```python
from build123d import *

# Parameters (mm, degrees)
SKETCH2_R            = 71
BOSS_EXTRUDE1_DEPTH  = 11
SKETCH12_R           = 57.5
SKETCH12_R_2         = 23.75
CUT_EXTRUDE8_DEPTH   = 1
CUT_EXTRUDE9_START   = -10
SKETCH10_R           = 85
SKETCH10_R_2         = 81
CUT_EXTRUDE9_DEPTH   = 10
SKETCH14_R           = 57.5
SKETCH14_R_2         = 23.75
BOSS_EXTRUDE2_DEPTH  = 1
SKETCH15_R           = 81
BOSS_EXTRUDE3_DEPTH  = 4
SKETCH16_R           = 57.5
SKETCH16_R_2         = 23.75
CUT_EXTRUDE11_DEPTH  = 2
SKETCH17_W           = 29
SKETCH17_H           = 10.11
SKETCH17_H_2         = 35.11
BOSS_EXTRUDE4_DEPTH  = 3
SKETCH19_R           = 80.970867582
BOSS_EXTRUDE5_DEPTH  = 2
BOSS_EXTRUDE6_START  = -3
SKETCH20_R           = 80.970867582
BOSS_EXTRUDE6_DEPTH  = 3
SKETCH21_W           = 29
SKETCH21_H           = 45.22
BOSS_EXTRUDE7_DEPTH  = 4
BOSS_EXTRUDE9_DEPTH  = 5
CUT_EXTRUDE12_START  = -5
SKETCH26_R           = 80.970867582
CUT_EXTRUDE12_DEPTH  = 5
BOSS_EXTRUDE10_START = -4
SKETCH27_R           = 80.970867582
BOSS_EXTRUDE10_DEPTH = 4
CUT_EXTRUDE15_REACH  = 120.043
SKETCH28_R           = 80.970867582
SKETCH28_R_2         = 80


with BuildPart() as part:
    # Sketch1 → Revolve1 (revolve)
    with BuildSketch(Plane.XY, mode=Mode.PRIVATE) as revolve1_sk:
        Polygon((0, 12), (0, 15), (85, 15), (85, 10.5), (84, 10.5), (77, 3.5), (77, 0), (71, 0), (71, 12), (23.75, 12), (23.75, -7.5), (21.25, -7.5), (21.25, 6), (6.5, 6), (6.5, 9), (0, 9), align=None)
    revolve(revolve1_sk.sketch.rotate(Axis((0, 12, 0), (0, -1, 0)), 180), axis=Axis((0, 12, 0), (0, -1, 0)))

    # Sketch2 → Boss-Extrude1 (add)
    with BuildSketch(Plane.XZ.offset(-12)):
        with Locations(Location((0, 0, 0), (0, 0, 180))):
            Circle(SKETCH2_R)
        Polygon((0, 70.292395274), (-60.875, 35.146197637), (-60.875, -35.146197637), (0, -70.292395274), (60.875, -35.146197637), (60.875, 35.146197637), align=None, mode=Mode.SUBTRACT)
    extrude(amount=BOSS_EXTRUDE1_DEPTH)

    # Sketch12 → Cut-Extrude8 (cut)
    with BuildSketch(Plane.XZ.offset(-12)):
        Circle(SKETCH12_R)
        with Locations(Location((0, 0, 0), (0, 0, 180))):
            Circle(SKETCH12_R_2, mode=Mode.SUBTRACT)
    extrude(amount=-CUT_EXTRUDE8_DEPTH, mode=Mode.SUBTRACT)

    # Sketch10 → Cut-Extrude9 (cut)
    with BuildSketch(Plane(origin=(0, 15, 0), x_dir=(1, 0, 0), z_dir=(0, 1, 0)).offset(CUT_EXTRUDE9_START)):
        Circle(SKETCH10_R)
        with Locations(Location((0, 0, 0), (0, 0, 180))):
            Circle(SKETCH10_R_2, mode=Mode.SUBTRACT)
    extrude(amount=CUT_EXTRUDE9_DEPTH, mode=Mode.SUBTRACT)

    # Sketch14 → Boss-Extrude2 (add)
    with BuildSketch(Plane(origin=(0, 13, 0), x_dir=(-1, 0, 0), z_dir=(0, -1, 0))):
        with Locations(Location((0, 0, 0), (0, 0, 180))):
            Circle(SKETCH14_R)
        Circle(SKETCH14_R_2, mode=Mode.SUBTRACT)
    extrude(amount=-BOSS_EXTRUDE2_DEPTH)

    # Sketch15 → Boss-Extrude3 (add)
    with BuildSketch(Plane(origin=(0, 15, 0), x_dir=(1, 0, 0), z_dir=(0, 1, 0))):
        with Locations(Location((0, 0, 0), (0, 0, 180))):
            Circle(SKETCH15_R)
    extrude(amount=BOSS_EXTRUDE3_DEPTH)

    # Sketch16 → Cut-Extrude11 (cut)
    with BuildSketch(Plane.XZ.offset(-13)):
        Circle(SKETCH16_R)
        with Locations(Location((0, 0, 0), (0, 0, 180))):
            Circle(SKETCH16_R_2, mode=Mode.SUBTRACT)
    extrude(amount=-CUT_EXTRUDE11_DEPTH, mode=Mode.SUBTRACT)

    # Sketch17 → Boss-Extrude4 (add)
    with BuildSketch(Plane(origin=(0, 19, 0), x_dir=(1, 0, 0), z_dir=(0, 1, 0))):
        with Locations((-48.833648901, -5.055)):
            Rectangle(SKETCH17_W, SKETCH17_H)
        with Locations((-48.833648901, 17.555)):
            Rectangle(SKETCH17_W, SKETCH17_H_2)
        with Locations((48.416351099, -5.055)):
            Rectangle(SKETCH17_W, SKETCH17_H)
        with Locations((48.416351099, 17.555)):
            Rectangle(SKETCH17_W, SKETCH17_H_2)
    extrude(amount=BOSS_EXTRUDE4_DEPTH)

    # Sketch19 → Boss-Extrude5 (add)
    with BuildSketch(Plane(origin=(0, 19, 0), x_dir=(1, 0, 0), z_dir=(0, 1, 0))):
        with Locations(Location((0, 0, 0), (0, 0, 180))):
            Circle(SKETCH19_R)
    extrude(amount=BOSS_EXTRUDE5_DEPTH)

    # Sketch20 → Boss-Extrude6 (add)
    with BuildSketch(Plane(origin=(0, 21, 0), x_dir=(1, 0, 0), z_dir=(0, 1, 0)).offset(BOSS_EXTRUDE6_START)):
        with Locations(Location((0, 0, 0), (0, 0, 180))):
            Circle(SKETCH20_R)
    extrude(amount=BOSS_EXTRUDE6_DEPTH)

    # Sketch21 → Boss-Extrude7 (add)
    with BuildSketch(Plane(origin=(0, 22, 0), x_dir=(1, 0, 0), z_dir=(0, 1, 0))):
        with Locations((48.416351099, 12.5)):
            Rectangle(SKETCH21_W, SKETCH21_H)
        with Locations((-48.833648901, 12.5)):
            Rectangle(SKETCH21_W, SKETCH21_H)
    extrude(amount=BOSS_EXTRUDE7_DEPTH)

    # Sketch22 → Boss-Extrude9 (add)
    with BuildSketch(Plane(origin=(0, 21, 0), x_dir=(1, 0, 0), z_dir=(0, 1, 0))):
        Polygon((48.416351099, 35.11), (37.416351099, 35.11), (37.416351099, 50.11), (59.416351099, 50.11), (59.416351099, 35.11), align=None)
    extrude(amount=BOSS_EXTRUDE9_DEPTH)

    # Sketch26 → Cut-Extrude12 (cut)
    with BuildSketch(Plane(origin=(0, 26, 0), x_dir=(1, 0, 0), z_dir=(0, 1, 0)).offset(CUT_EXTRUDE12_START)):
        with Locations(Location((0, 0, 0), (0, 0, 180))):
            Circle(SKETCH26_R)
    extrude(amount=CUT_EXTRUDE12_DEPTH, mode=Mode.SUBTRACT)

    # Sketch27 → Boss-Extrude10 (add)
    with BuildSketch(Plane(origin=(0, 21, 0), x_dir=(1, 0, 0), z_dir=(0, 1, 0)).offset(BOSS_EXTRUDE10_START)):
        with Locations(Location((0, 0, 0), (0, 0, 180))):
            Circle(SKETCH27_R)
    extrude(amount=BOSS_EXTRUDE10_DEPTH)

    # Cut-Extrude15: up to this cone (the profile starts inside it)
    cut_extrude15_end = Plane(origin=(0, 21, 0), z_dir=(0, 1, 0)).offset(-94.499999) * Cone(1e-06, 309.543, 309.542999, align=(Align.CENTER, Align.CENTER, Align.MIN), mode=Mode.PRIVATE)
    # Sketch28 → Cut-Extrude15 (cut, up to the surface)
    with BuildSketch(Plane(origin=(0, 21, 0), x_dir=(1, 0, 0), z_dir=(0, 1, 0)), mode=Mode.PRIVATE) as cut_extrude15_sk1:
        Circle(SKETCH28_R)
        with Locations(Location((0, 0, 0), (0, 0, 180))):
            Circle(SKETCH28_R_2, mode=Mode.SUBTRACT)
    cut_extrude15_tool1 = extrude(cut_extrude15_sk1.sketch, amount=-CUT_EXTRUDE15_REACH, mode=Mode.PRIVATE) & cut_extrude15_end
    add(cut_extrude15_tool1.solids().sort_by_distance((-80.741847, 21, 0))[0], mode=Mode.SUBTRACT)


with BuildPart() as body_2:
    # of the pieces the cut leaves, the one that is kept (cut_extrude15_keep)
    add(part.part.solids().sort_by_distance((-80, 6.5, 0))[0])


solid = body_2.part
```
Model file for the job. Use its own axes, mm. A direction names the side the tool comes from. Round coordinates to 2 decimals unless told otherwise and drop trailing zeros. Loops run counter-clockwise (first coordinate to the right, second up) from the corner with the lowest first, then second, coordinate; pieces in that order, holes last. Notation, with made-up numbers: M 27.5,12 L 85.5,12 A19 cw 85.5,29 Z; hole C -6,-39.75 d6. An arc over 180 degrees is marked long. Put each result on its own line as item: value. Start each with the question number.
Item 1: 3-axis set-ups, long thin cutter, end or side, ignore diameter. For faces 4 (the face through (18, -7.5, 12)), 5 (the face through (5.149, 3.592, 23.185)): which of +Z, -Z, +X, -X, +Y, -Y reach the whole face in a straight line?
Item 2: Mould opens along Z. For faces 1 (the face through (0, 9, 0)), 2 (the face through (1, 21, 1)), 3 (the face through (-73.583, 3.646, -23.172)) say: released by +Z, released by -Z, zero draft, split by the parting line, or undercut.
Item 3: Drop flat-ended pins along their axis: P1, Ø3.5, axis at y = 8, z = -14, coming from the -X side; P2, Ø1.5, axis at x = 34.5, y = 5, coming from the -Z side; P3, Ø1, axis at x = -20, y = 6, coming from the +Z side. Give the stop position or say it passes through.
Item 4: Cut at B-B (y = 17). List the corners of the cut face in (x, z).
Item 5: Drill centre lines: line 1 along Z through (x, y) = (0, 0.35); line 2 along Z through (x, y) = (0, 8.1); line 3 along X through (y, z) = (5, 10.5) (3 decimals). Where is each one in solid material? Low to high.
Answer block:
1. face 4: +Z, -Z, +X, -X, -Y
1. face 5: -Y
2. face 1: undercut
2. face 2: zero draft
2. face 3: split by the parting line
3. P1: x = -79.06
3. P2: z = -71.42
3. P3: z = 77.48
4. outline: C 0,0 d160
5. line 1: -77 to -71, -23.75 to -21.25, 21.25 to 23.75, 71 to 77
5. line 2: -80 to -70.29, -23.75 to -6.5, 6.5 to 23.75, 70.29 to 80
5. line 3: -77.795 to -60.875, -21.303 to -18.475, 18.475 to 21.303, 60.875 to 77.795
